Geometry check sheet. Reference: the model listing, model coordinates, mm. Round coordinates to 2 decimals unless told otherwise and drop trailing zeros. Write each loop counter-clockwise with the first axis right and the second up, starting at its lowest first coordinate (ties: lowest second). Pieces come first, ordered by that corner, then holes.
from build123d import *

# Parameters (mm, degrees)
SKETCH_1_W               = 150
SKETCH_1_H               = 105
SKETCH_1_R               = 2
EXTRUDE_1_DEPTH          = 4
SKETCH_2_W               = 270
SKETCH_2_H               = 170
EXTRUDE_2_DEPTH          = 4
CUT_EXTRUDE_2_DEPTH      = 193.860701025
CUT_EXTRUDE_2_DEPTH_BACK = 193.860701025
SKETCH_3_R               = 2
FILLET_1_R               = 6
CUT_EXTRUDE_3_DEPTH      = 193.736218703
CUT_EXTRUDE_3_DEPTH_BACK = 193.736218703
SKETCH_4_R               = 1.5
CUT_EXTRUDE_4_DEPTH      = 193.736218703
CUT_EXTRUDE_4_DEPTH_BACK = 193.736218703
SKETCH_5_W               = 57.583887605
SKETCH_5_H               = 127.518164053
FILLET_2_R               = 6
FILLET_3_R               = 5


with BuildPart() as part:
    # 草图1 → 凸台-拉伸1 (new body)
    with BuildSketch(Plane(origin=(0, 0, 0), x_dir=(1, 0, 0), z_dir=(0, 1, 0))):
        with Locations((0, 52.5)):
            Rectangle(SKETCH_1_W, SKETCH_1_H)
        with Locations(Location((-37.5, 90, 0), (0, 0, 270))):
            Circle(SKETCH_1_R, mode=Mode.SUBTRACT)
        with Locations(Location((-37.5, 15, 0), (0, 0, 270))):
            Circle(SKETCH_1_R, mode=Mode.SUBTRACT)
        with Locations(Location((37.5, 15, 0), (0, 0, 270))):
            Circle(SKETCH_1_R, mode=Mode.SUBTRACT)
        with Locations(Location((37.5, 90, 0), (0, 0, 270))):
            Circle(SKETCH_1_R, mode=Mode.SUBTRACT)
    extrude(amount=EXTRUDE_1_DEPTH)

    # 草图2 → 凸台-拉伸2 (add)
    with BuildSketch(Plane.XZ):
        with Locations((0, -52.5)):
            Rectangle(SKETCH_2_W, SKETCH_2_H)
    extrude(amount=EXTRUDE_2_DEPTH)

    # 草图3 → 切除-拉伸2 (cut, two sides: drawn at the far end of the back side and taken through both)
    with BuildSketch(Plane(origin=(0, 4, 0), x_dir=(1, 0, 0), z_dir=(0, 1, 0)).offset(-CUT_EXTRUDE_2_DEPTH_BACK)):
        with Locations(Location((-37.5, 90, 0), (0, 0, 270))):
            Circle(SKETCH_3_R)
        with Locations(Location((37.5, 90, 0), (0, 0, 270))):
            Circle(SKETCH_3_R)
        with Locations(Location((-37.5, 15, 0), (0, 0, 270))):
            Circle(SKETCH_3_R)
        with Locations(Location((37.5, 15, 0), (0, 0, 270))):
            Circle(SKETCH_3_R)
    extrude(amount=CUT_EXTRUDE_2_DEPTH + CUT_EXTRUDE_2_DEPTH_BACK, mode=Mode.SUBTRACT)

    # 圆角1
    fillet_1_edges = [part.edges().sort_by_distance(p)[0] for p in [
        (135, -2, -137.5),
        (135, -2, 32.5),
        (-135, -2, 32.5),
        (-135, -2, -137.5),
    ]]
    fillet(fillet_1_edges, radius=FILLET_1_R)

    # 草图4 → 切除-拉伸3 (cut, two sides: drawn at the far end of the back side and taken through both)
    with BuildSketch(Plane(origin=(0, 0, 0), x_dir=(1, 0, 0), z_dir=(0, 1, 0)).offset(-CUT_EXTRUDE_3_DEPTH_BACK)):
        with Locations(Location((-129, 52.5, 0), (0, 0, 270))):
            Circle(SKETCH_4_R)
        with Locations(Location((-129, -26.5, 0), (0, 0, 270))):
            Circle(SKETCH_4_R)
        with Locations(Location((-56, -26.5, 0), (0, 0, 270))):
            Circle(SKETCH_4_R)
        with Locations(Location((56, -26.5, 0), (0, 0, 270))):
            Circle(SKETCH_4_R)
        with Locations(Location((129, -26.5, 0), (0, 0, 270))):
            Circle(SKETCH_4_R)
        with Locations(Location((129, 52.5, 0), (0, 0, 270))):
            Circle(SKETCH_4_R)
        with Locations(Location((56, 131.5, 0), (0, 0, 270))):
            Circle(SKETCH_4_R)
        with Locations(Location((129, 131.5, 0), (0, 0, 270))):
            Circle(SKETCH_4_R)
        with Locations(Location((-56, 131.5, 0), (0, 0, 270))):
            Circle(SKETCH_4_R)
        with Locations(Location((-129, 131.5, 0), (0, 0, 270))):
            Circle(SKETCH_4_R)
    extrude(amount=CUT_EXTRUDE_3_DEPTH + CUT_EXTRUDE_3_DEPTH_BACK, mode=Mode.SUBTRACT)

    # 草图5 → 切除-拉伸4 (cut, two sides: drawn at the far end of the back side and taken through both)
    with BuildSketch(Plane(origin=(0, 0, 0), x_dir=(1, 0, 0), z_dir=(0, 1, 0)).offset(-CUT_EXTRUDE_4_DEPTH_BACK)):
        with Locations((-106.208056197, 54.041877238)):
            Rectangle(SKETCH_5_W, SKETCH_5_H)
    extrude(amount=CUT_EXTRUDE_4_DEPTH + CUT_EXTRUDE_4_DEPTH_BACK, mode=Mode.SUBTRACT)

    # 圆角2
    fillet_2_edges = [part.edges().sort_by_distance(p)[0] for p in [
        (-135, -2, 9.717204788),
        (-77.416112395, -2, -117.800959265),
        (-135, -2, -117.800959265),
        (-77.416112395, -2, 9.717204788),
    ]]
    fillet(fillet_2_edges, radius=FILLET_2_R)

    # 圆角3
    fillet_3_edges = [part.edges().sort_by_distance(p)[0] for p in [
        (-75, 2, -105),
        (75, 2, -105),
        (75, 2, 0),
        (-75, 2, 0),
    ]]
    fillet(fillet_3_edges, radius=FILLET_3_R)


solid = part.part
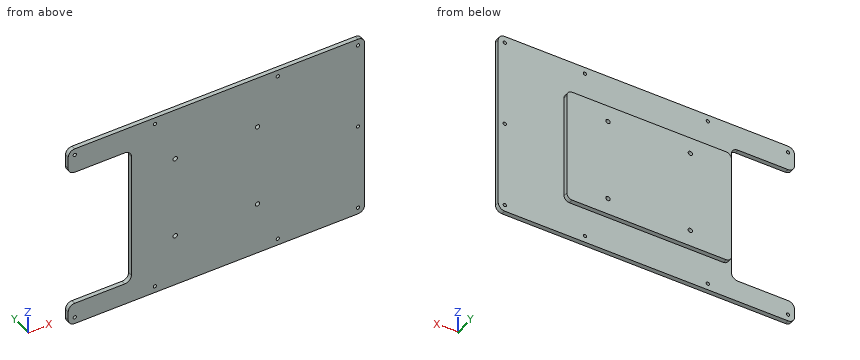
1. Depth check by flat-ended pin: pin 1 Ø8 at (x, z) = (-100, 4.5) entering from -Y; pin 2 Ø5 at (x, z) = (129, -52.5) entering from +Y; pin 3 Ø1.2 at (y, z) = (2, -69) entering from -X; pin 4 Ø4 at (y, z) = (-1, -65) entering from -X. Enter the tip coordinate at first touch or a pass-through.
2. Section check D-D (x = 115.5). Record the cut outline in (y, z).
3. Section check A-A (x = -113). Record the cut outline in (y, z).
4. Scan lines: line 1 along Z through (x, y) = (129, -1.2); line 2 along Z through (x, y) = (56, -1.1); line 3 along Z through (x, y) = (37.5, -0.25). Record each from-to range of solid material in increasing order.
5. Section check C-C (x = -21). Record the cut outline in (y, z).
6. Section check B-B (y = -2). State how many separate pieces and enclosed holes the cut face has, plus the area to 3 significant figures.
Results below:
1. pin 1: passes through
1. pin 2: stops at y = 0
1. pin 3: stops at x = -75
1. pin 4: stops at x = -77.42
2. outline: (-4, -137.5) - (0, -137.5) - (0, 32.5) - (-4, 32.5) - close
3. outline: (-4, -137.5) - (0, -137.5) - (0, -117.8) - (-4, -117.8) - close; (-4, 9.72) - (0, 9.72) - (0, 32.5) - (-4, 32.5) - close
4. line 1: z = -137.5 to -133, -130 to -54, -51 to 25, 28 to 32.5
4. line 2: z = -137.5 to -133, -130 to 25, 28 to 32.5
4. line 3: z = -137.5 to -92, -88 to -17, -13 to 32.5
5. outline: (-4, -137.5) - (0, -137.5) - (0, -105) - (4, -105) - (4, 0) - (0, 0) - (0, 32.5) - (-4, 32.5) - close
6. separate pieces: 1
6. enclosed holes: 13
6. area: 38,400 mm2
